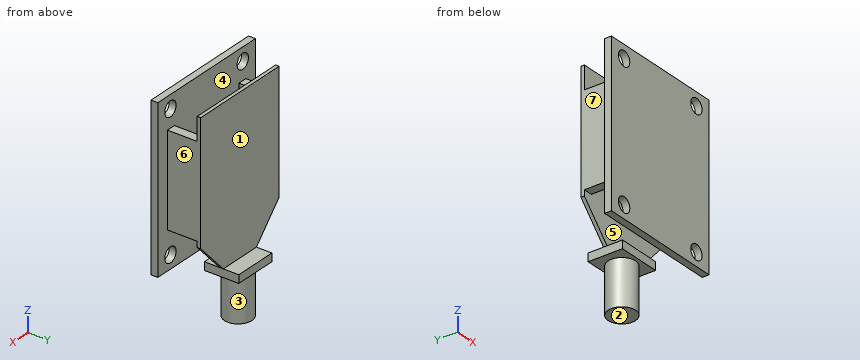
Autodesk Inventor part; units mm, degrees
ref_plane "YZ Plane" through (0, 0, 0) normal (1, 0, 0) x (0, 1, 0)
ref_plane "XZ Plane" through (0, 0, 0) normal (0, 1, 0) x (-1, 0, 0)
ref_plane "XY Plane" through (0, 0, 0) normal (0, 0, 1) x (1, 0, 0)
sketch "Sketch2" plane through (0, 0, 0) normal (0, 1, 0) x (-1, 0, 0)
  line L0 (-14.224, 17.78) -> (14.224, 17.78)
  line L1 (14.224, 17.78) -> (14.224, -17.78)
  line L2 (14.224, -17.78) -> (-14.224, -17.78)
  line L3 (-14.224, -17.78) -> (-14.224, 17.78)
  circle A0 centre (-10.541, 14.859) radius 1.651
  circle A1 centre (-10.541, -14.859) radius 1.651
  line L4 (0, 13.208) -> (0, -8.1739) construction
  circle A2 centre (10.541, 14.859) radius 1.651
  circle A3 centre (10.541, -14.859) radius 1.651
  point P0 (0, 0)
  dimension "d0" = 28.448
  dimension "d1" = 35.56
  dimension "d2" = 14.224
  dimension "d3" = 17.78
  dimension "d4" = 3.302
  dimension "d5" = 1.27
  dimension "d6" = 2.032
  dimension "d7" = 3.302
  dimension "d8" = 1.27
  dimension "d9" = 2.032
extrude "Extrusion1" add sketch "Sketch2" along normal blind 1.524
sketch "Sketch3" plane through (0, 1.524, 0) normal (0, 1, 0) x (1, 0, 0)
  line L0 (-14.224, -17.78) -> (-14.224, 17.78)
  line L1 (-14.224, 17.78) -> (14.224, 17.78)
  line L2 (-11.43, 9.398) -> (-9.398, 9.398)
  line L3 (-9.398, 9.398) -> (-9.398, -10.922)
  line L4 (-9.398, -10.922) -> (-11.43, -10.922)
  line L5 (-11.43, -10.922) -> (-11.43, 9.398)
  line L6 (0, 9.398) -> (0, -9.2858) construction
  line L7 (11.43, 9.398) -> (9.398, 9.398)
  line L8 (9.398, 9.398) -> (9.398, -10.922)
  line L9 (9.398, -10.922) -> (11.43, -10.922)
  line L10 (11.43, -10.922) -> (11.43, 9.398)
  point P0 (0, 0)
  dimension "d12" = 2.032
  dimension "d13" = 20.32
  dimension "d14" = 2.794
  dimension "d15" = 8.382
extrude "Extrusion2" add sketch "Sketch3" along normal blind 6.604
sketch "Sketch4" plane through (0, 8.128, 0) normal (0, 1, 0) x (1, 0, 0)
  line L0 (-9.398, 9.398) -> (-9.398, -10.922)
  line L1 (-11.43, 9.398) -> (-9.398, 9.398)
  line L2 (-11.43, -10.922) -> (-11.43, 9.398)
  line L3 (-9.398, -10.922) -> (-11.43, -10.922)
  line L4 (11.43, 10.668) -> (11.43, -16.002)
  line L5 (11.43, -16.002) -> (-11.43, -16.002)
  line L6 (-11.43, -16.002) -> (-11.43, 10.668)
  line L7 (-11.43, 10.668) -> (-4.826, 17.78)
  line L8 (-4.826, 17.78) -> (4.826, 17.78)
  line L9 (-14.224, -17.78) -> (-14.224, 17.78)
  line L10 (4.826, 17.78) -> (11.43, 10.668)
  line L11 (-11.43, 5.9569) -> (-11.43, -5.9458) construction
  line L12 (14.224, 17.78) -> (14.224, -17.78) construction
  point P0 (0, 0)
  dimension "d18" = 2.794
  dimension "d19" = 2.794
  dimension "d20" = 5.08
  dimension "d21" = 9.652
  dimension "d23" = 26.67
  dimension "d24" = 42.879
  dimension "d25" = 137.121
  dimension "d26" = 16.8789
  dimension "d27" = 4.9762
extrude "Extrusion3" add sketch "Sketch4" along normal blind 0.762
sketch "Sketch5" plane through (4.826, 8.128, -17.78) normal (0, 0, -1) x (-1, 0, 0)
  line L0 (9.652, 0.762) -> (0, 0.762)
  line L1 (0, 0) -> (0, 0.762)
  line L2 (9.652, 0) -> (9.652, 0.762)
  line L3 (0, 4.191) -> (9.652, 4.191)
  line L4 (9.652, 4.191) -> (9.652, -3.429)
  line L5 (9.652, -3.429) -> (0, -3.429)
  line L6 (0, -3.429) -> (0, 4.191)
  point P0 (4.826, -8.128)
  point P1 (0, 0.381)
  point P2 (9.652, 0.381)
  dimension "d30" = 7.62
  dimension "d31" = 3.429
extrude "Extrusion4" add sketch "Sketch5" along normal blind 1.778
sketch "Sketch6" plane through (4.826, 8.128, -19.558) normal (0, 0, -1) x (-1, 0, 0)
  circle A0 centre (4.826, 0.381) radius 3.048
  line L0 (0, 4.191) -> (9.652, -3.429) construction
  point P0 (4.826, -8.128)
  point P1 (4.826, 0.381)
  dimension "d34" = 6.096
extrude "Extrusion5" add sketch "Sketch6" along normal blind 10.033
properties part number "XBee"
Geometry: final body of the model. Coordinates: model frame, mm. Face numbers are marked on the shaded views. A direction names the side the tool comes from. Round coordinates to 2 decimals unless told otherwise and drop trailing zeros. Order: outer loops, then holes, each group sorted by start corner. A loop starts at its lowest first (then second) coordinate and runs counter-clockwise, first axis right, second up. Notation, with made-up numbers: (59, -14.5) -> (103, -14.5) arc R5 cw to (103, -10.5) -> close; hole circle Ø6 at (24.5, 78). An arc over 180 degrees is marked (long way). Use one line per item in the form item = value.
(1) Draft query along X for the marked faces 4, 5, 6 and 7. Return one class per face: pulls with the +X half, pulls with the -X half, needs draft (parallel to the pull), parting line crosses it, or undercut.
Results list:
face_4 = undercut
face_5 = undercut
face_6 = pulls with the +X half
face_7 = pulls with the -X half
(2) First-contact query: pin 1 Ø3 at (x, y) = (6, 7.5) entering from -Z; pin 2 Ø1.4 at (y, z) = (7.5, -18.5) entering from +X; pin 3 Ø6 at (x, y) = (-8, 9.5) entering from +Z. Flat tips, straight axial feed; report the tip coordinate or a pass-through.
Results list:
pin_1 = -19.56
pin_2 = 4.83
pin_3 = 16
(3) Section C-C on x = 0. Return loops of the section in (y, z), and give its area (3 significant figures).
Results list:
outline = (0, -17.78) -> (1.52, -17.78) -> (1.52, 17.78) -> (0, 17.78) -> close; (4.7, -19.56) -> (5.46, -19.56) -> (5.46, -29.59) -> (11.56, -29.59) -> (11.56, -19.56) -> (12.32, -19.56) -> (12.32, -17.78) -> (8.89, -17.78) -> (8.89, 16) -> (8.13, 16) -> (8.13, -17.78) -> (4.7, -17.78) -> close
area = 155 mm^2
(4) Section A-A on y = 2.5. Return loops of the section in (x, z), and give its area (3 significant figures).
Results list:
outline = (-11.43, -9.4) -> (-9.4, -9.4) -> (-9.4, 10.92) -> (-11.43, 10.92) -> close; (9.4, -9.4) -> (11.43, -9.4) -> (11.43, 10.92) -> (9.4, 10.92) -> close
area = 82.6 mm^2
(5) Access query for the marked faces 1, 2 and 3. Directions: +Z, -Z, +X, -X, +Y, -Y. A direction counts if a zero-diameter tool reaches every point of the face in a straight line with its end or side. Return the directions, or none.
Results list:
face_1 = +Z, +X, -X, +Y
face_2 = -Z, +X, -X, +Y, -Y
face_3 = -Z
(6) Section B-B on z = 1. Return loops of the section in (x, y).
Results list:
outline = (-14.22, 0) -> (14.22, 0) -> (14.22, 1.52) -> (11.43, 1.52) -> (11.43, 8.89) -> (-11.43, 8.89) -> (-11.43, 1.52) -> (-14.22, 1.52) -> close; hole (-9.4, 1.52) -> (9.4, 1.52) -> (9.4, 8.13) -> (-9.4, 8.13) -> close
(7) Section D-D on z = -10. Return loops of the section in (x, y), and give its area (3 significant figures).
Results list:
outline = (-14.22, 0) -> (14.22, 0) -> (14.22, 1.52) -> (-14.22, 1.52) -> close; (-11.43, 8.13) -> (11.43, 8.13) -> (11.43, 8.89) -> (-11.43, 8.89) -> close
area = 60.8 mm^2
(8) Ray query, probe 1 along X at (y, z) = (3.25, -2); probe 2 along Y at (x, z) = (-1.25, -5); probe 3 along Z at (x, y) = (-1, 8). Return the intervals inside material, ascending. Write a range as [from, to].
Results list:
probe_1 = [-11.43, -9.4], [9.4, 11.43]
probe_2 = [0, 1.52], [8.13, 8.89]
probe_3 = [-29.59, -17.78]
